Here's how the part is built. I have some questions about the finished solid (model axes, mm). A direction names the side the tool comes from. Coordinates: 2 decimals unless noted, no trailing zeros. Write each loop counter-clockwise with the first axis right and the second up, starting at its lowest first coordinate (ties: lowest second). Pieces come first, ordered by that corner, then holes.
```python
from build123d import *

# Parameters (mm, degrees)
PAD_DEPTH       = 15
SKETCH001_R     = 2.75
POCKET_DEPTH    = 25.001
SKETCH002_R     = 4.75
POCKET001_DEPTH = 20.001


with BuildPart() as part:
    # Sketch → Pad (new body)
    with BuildSketch(Plane.XY):
        with BuildLine():
            ThreePointArc((14.716063, 0), (0, 13.75), (-14.716063, 0))
            Line((-25.980762, 0), (-14.716063, 0))
            ThreePointArc((25.980762, 0), (0, 25), (-25.980762, 0))
            Line((14.716063, 0), (25.980762, 0))
        make_face()
    extrude(amount=PAD_DEPTH)

    # Sketch001 (on Face2 of Pad) → Pocket (cut, through all)
    with BuildSketch(Plane.XZ):
        with Locations((-19.125, 7.5)):
            Circle(SKETCH001_R)
        with Locations((19.125, 7.5)):
            Circle(SKETCH001_R)
    extrude(amount=-POCKET_DEPTH, mode=Mode.SUBTRACT)

    # Sketch002 (on DatumPlane) → Pocket001 (cut, through all)
    with BuildSketch(Plane.XZ.offset(-5)):
        with Locations((-19.125, 7.5)):
            Circle(SKETCH002_R)
        Polygon((19.125, 2.592523), (23.375, 5.046261), (23.375, 9.953739), (19.125, 12.407477), (14.875, 9.953739), (14.875, 5.046261), align=None)
    extrude(amount=-POCKET001_DEPTH, mode=Mode.SUBTRACT)


solid = part.part
```
1) Imagine slicing it at D-D on y = 11.5. Please give me the cut outline in (x, z) (3 decimals), then the cut area to 3 significant figures.
Values follow:
outline: (-22.798, 0) - (-7.83, 0) - (-7.83, 15) - (-22.798, 15) - (-22.798, 10.512) arc R4.75 cw (long way) to (-22.798, 4.488) - close; (7.83, 0) - (22.798, 0) - (22.798, 4.713) - (19.125, 2.593) - (14.875, 5.046) - (14.875, 9.954) - (19.125, 12.407) - (22.798, 10.287) - (22.798, 15) - (7.83, 15) - close
area: 323 mm2
2) On a 3-axis mill with a long thin cutter (end or side, diameter ignored), from which of +Z, -Z, +X, -X, +Y, -Y can I reach the whole of each face in a straight line? I mean faces 4 (the face through (16.97, 12.555, 3.837)), 5 (the face through (-22, 0, 9)). Say none if no direction works.
Values follow:
face 4: +Y
face 5: +Z, -Z, +X, -X, -Y
3) I need wall thicknesses on probe 1 along X at (y, z) = (7, 11.25); probe 2 along X at (y, z) = (8, 4.5); probe 3 along Z at (x, y) = (-21.5, 8.25). Which ranges of each line are inside material? Lowest first, please.
Values follow:
probe 1: x = -24.74 to -22.04, -16.21 to -12.39, 12.39 to 17.12, 21.13 to 24.74
probe 2: x = -24.39 to -22.81, -15.44 to -11.69, 11.69 to 15.82, 22.43 to 24.39
probe 3: z = 0 to 3.39, 11.61 to 15
4) Will these pins go through, and if not, where does the flat tip stop? pin 1 (4 mm diameter, centred on y = 9.5, z = 9.5, fed in from +X); pin 2 (4 mm diameter, centred on x = 20.5, z = 7.5, fed in from +Y); pin 3 (2 mm diameter, centred on x = -4, z = 11, fed in from -Y).
Values follow:
pin 1: stops at x = 24.57
pin 2: stops at y = 5
pin 3: stops at y = 12.88
5) We'd pull the mould along Z, two halves only. Please class faces 1 (the face through (16.94, 2.46, 5.83)), 2 (the face through (22, 0, 9)), 3 (the face through (0, 15, 15)): pulls with the +Z half, pulls with the -Z half, needs draft (parallel to the pull), parting line crosses it, or undercut.
Values follow:
face 1: undercut
face 2: needs draft
face 3: pulls with the +Z half
6) Imagine slicing it at B-B on y = 1.5. Please give me the cut outline in (x, z) (3 decimals).
Values follow:
outline: (-25.88, 0) - (-14.537, 0) - (-14.537, 15) - (-25.88, 15) - close; (14.537, 0) - (25.88, 0) - (25.88, 15) - (14.537, 15) - close; hole circle Ø5.5 at (-19.125, 7.5); hole circle Ø5.5 at (19.125, 7.5)
7) Imagine slicing it at C-C on x = -18. Please give me the cut outline in (y, z), then the cut area to 3 significant figures.
Values follow:
outline: (0, 0) - (17.76, 0) - (17.76, 2.89) - (5, 2.89) - (5, 4.99) - (0, 4.99) - close; (0, 10.01) - (5, 10.01) - (5, 12.11) - (17.76, 12.11) - (17.76, 15) - (0, 15) - close
area: 124 mm2
8) Imagine slicing it at A-A on z = 8.5. Count the separate pieces of the cut face and the enclosed holes in it, then the cut area to 3 significant figures.
Values follow:
separate pieces: 3
enclosed holes: 0
area: 448 mm2
